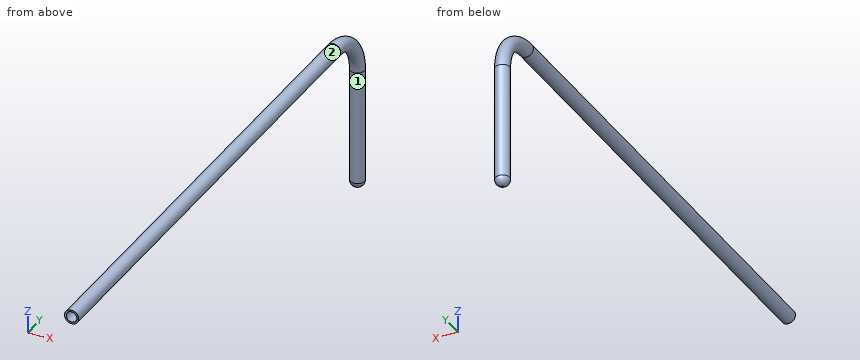
Autodesk Inventor part; units mm, degrees
ref_plane "YZ Plane" through (0, 0, 0) normal (1, 0, 0) x (0, 1, 0)
ref_plane "XZ Plane" through (0, 0, 0) normal (0, 1, 0) x (-1, 0, 0)
ref_plane "XY Plane" through (0, 0, 0) normal (0, 0, 1) x (1, 0, 0)
sketch "Sketch1" plane through (0, 0, 0) normal (0, 1, 0) x (-1, 0, 0)
  circle A0 centre (0, 0) radius 3.9688
  circle A1 centre (0, 0) radius 2.9688
  dimension "d0" = 7.9375
  dimension "d4" = 1
sketch "Sketch2" plane through (0, 0, 0) normal (1, 0, 0) x (0, 1, 0)
  line L0 (0, 0) -> (275, 0)
  line L1 (300, -25) -> (300, -90)
  arc A0 (300, -25) -> (275, 0) centre (275, -25) ccw
  point P0 (300, 0)
  dimension "d1" = 300
  dimension "d2" = 90
  dimension "d3" = 25
sweep "Sweep1" add profiles "Sketch1" path "Sketch2"
sketch "Sketch3" plane through (0, 0, 0) normal (1, 0, 0) x (0, 1, 0)
  line L0 (296.0312, -90) -> (303.9688, -90)
  arc A0 (300.25, -93.9609) -> (299.75, -93.9609) centre (300, -90) ccw
  line L1 (300, -90) -> (300, -93.9688)
  line L2 (300.25, -90) -> (300.25, -93.9609)
  line L3 (299.75, -90) -> (299.75, -93.9609)
  point P0 (0, 0)
  point P1 (300.25, -96.7948)
  point P2 (299.75, -96.7948)
  dimension "d7" = 0.25
revolve "Revolution1" add sketch "Sketch3" angle 360 about axis through (0, 300, -90) along (0, 0, -1) contours A0 L2 L0
properties part number "Pitot Tube" material "Stainless Steel"
The model under review builds one solid part; all positions refer to its coordinate system, in mm. Face numbers are marked on the shaded views. A direction names the side the tool comes from. Round coordinates to 2 decimals unless told otherwise and drop trailing zeros. Order: outer loops, then holes, each group sorted by start corner. A loop starts at its lowest first (then second) coordinate and runs counter-clockwise, first axis right, second up. Notation, with made-up numbers: (-34.5, 36) -> (19.5, 36) arc R30 cw to (19.5, 67) -> close; hole circle Ø11 at (-28, 71). An arc over 180 degrees is marked (long way). Write item = value, one per line. Start each with the question number.
Item 1: Clearance check with flat-ended pins moving along their axes: pin 1 Ø4 at (x, y) = (1, 67) entering from -Z; pin 2 Ø3.5 at (x, z) = (0, 0) entering from +Y; pin 3 Ø4 at (x, z) = (0, -83.5) entering from -Y. State where each tip first meets the part, or that it passes through.
Item 2: For the marked faces 1 and 2, list the 3-axis set-ups (+Z, -Z, +X, -X, +Y, -Y) from which the entire face can be reached by the end or side of a thin tool; tool diameter is ignored.
Item 3: Consider section C-C on x = 1.75. Write out the cut boundary in (y, z), plus the area to 3 significant figures.
Item 4: For line 1 along X through (y, z) = (300, -37.5); line 2 along Z through (x, y) = (-0.25, 173); line 3 along Z through (x, y) = (-0.5, 233), list the stretches that pass through material, from the lowest coordinate up.
Item 5: Consider section B-B on z = -82. Write out the cut boundary in (x, y), plus the area to 3 significant figures.
Item 6: Consider section A-A on y = 271. Write out the cut boundary in (x, z), plus the area to 3 significant figures.
Conclusion:
q1.pin_1 = -3.97
q1.pin_2 = 292.28
q1.pin_3 = 296.03
q2.face_1 = -Z
q2.face_2 = -Y
q3.outline = (0, -3.56) -> (275, -3.56) arc R21.44 cw to (296.44, -25) -> (296.44, -90) arc R3.56 ccw to (303.56, -90) -> (303.56, -25) arc R28.56 ccw to (275, 3.56) -> (0, 3.56) -> (0, 2.4) -> (275, 2.4) arc R27.4 cw to (302.4, -25) -> (302.4, -90) -> (297.6, -90) -> (297.6, -25) arc R22.6 ccw to (275, -2.4) -> (0, -2.4) -> close
q3.area = 903 mm2
q4.line_1 = -3.97 to -2.97, 2.97 to 3.97
q4.line_2 = -3.96 to -2.96, 2.96 to 3.96
q4.line_3 = -3.94 to -2.93, 2.93 to 3.94
q5.outline = circle Ø7.94 at (0, 300); hole circle Ø5.94 at (0, 300)
q5.area = 21.8 mm2
q6.outline = circle Ø7.94 at (0, 0); hole circle Ø5.94 at (0, 0)
q6.area = 21.8 mm2
